Model file for the job. Use its own axes, mm. Face numbers are marked on the shaded views. A direction names the side the tool comes from. Coordinates: 2 decimals unless noted, no trailing zeros. Write each loop counter-clockwise with the first axis right and the second up, starting at its lowest first coordinate (ties: lowest second). Pieces come first, ordered by that corner, then holes. Notation, with made-up numbers: (80.5, -15) -> (88.5, -15) arc R16 ccw to (88.5, 8) -> close; hole circle Ø4 at (-5.5, 30.5). An arc over 180 degrees is marked (long way). Write item = value, one per line. Start each with the question number.
from build123d import *

# Parameters (mm, degrees)
BOSS_EXTRUDE1_DEPTH = 120
SKETCH2_R           = 40
BOSS_EXTRUDE2_DEPTH = 30
SKETCH4_R           = 60
BOSS_EXTRUDE3_DEPTH = 4
SHELL1_START        = 3
SHELL1_DEPTH        = 114
SHELL1_START_2      = 37.215764226
SHELL1_2_OUTLINE_R  = 37
SHELL1_2_DEPTH      = 34


with BuildPart() as part:
    # Sketch1 → Boss-Extrude1 (new body)
    with BuildSketch(Plane.XY):
        Polygon((40, 21.666666667), (-40, 75), (-40, -75), (40, -75), align=None)
    extrude(amount=BOSS_EXTRUDE1_DEPTH)

    # Sketch2 → Boss-Extrude2 (add)
    with BuildSketch(Plane(origin=(22.307692308, 33.461538462, 0), x_dir=(0, 0, -1), z_dir=(0.5547001962252291, 0.8320502943378437, 0))):
        with Locations(Location((-60, 26.810509484, 0), (0, 0, 90))):
            Circle(SKETCH2_R)
    extrude(amount=BOSS_EXTRUDE2_DEPTH)

    # Sketch4 → Boss-Extrude3 (add)
    with BuildSketch(Plane(origin=(38.948698194, 58.423047292, 0), x_dir=(0, 0, -1), z_dir=(0.5547001962252291, 0.8320502943378437, 0))):
        with Locations(Location((-60, 26.810509484, 0), (0, 0, 90))):
            Circle(SKETCH4_R)
    extrude(amount=BOSS_EXTRUDE3_DEPTH)

    # Shell1: read off the stored shape, not the designer's step
    # Shell1 outline → Shell1 (cut)
    with BuildSketch(Plane.XY.offset(SHELL1_START)):
        Polygon((-37, -72), (37, -72), (37, 20.061115391), (-37, 69.394448725), align=None)
    extrude(amount=SHELL1_DEPTH, mode=Mode.SUBTRACT)

    # Shell1 2 outline → Shell1 2 (cut)
    with BuildSketch(Plane(origin=(0, 0, 0), x_dir=(0.8320502943378438, -0.5547001962252289, 0), z_dir=(0.5547001962252289, 0.8320502943378438, 0)).offset(SHELL1_START_2)):
        with Locations((-26.810509484, -60)):
            Circle(SHELL1_2_OUTLINE_R)
    extrude(amount=SHELL1_2_DEPTH, mode=Mode.SUBTRACT)


solid = part.part
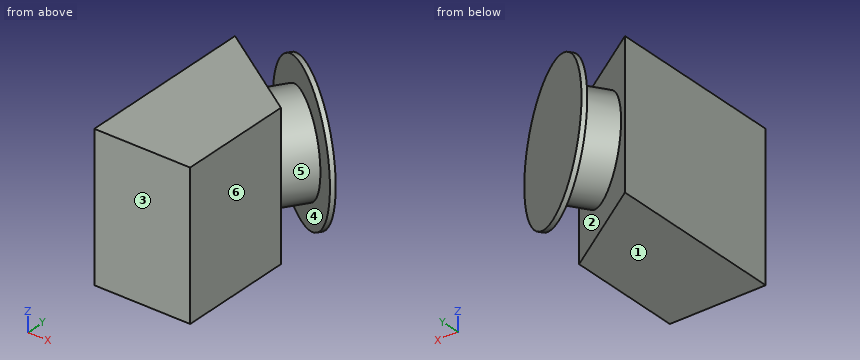
(1) Saw through at C-C (x = -26). State how many separate pieces and enclosed holes the cut face has, then the cut area to 3 significant figures.
(2) Saw through at A-A (z = 18). Give the cut face in (x, y).
(3) Saw through at D-D (z = 34). Give the cut face in (x, y).
(4) Drop flat-ended pins along their axis: pin 1 Ø22 at (x, y) = (0, 30) entering from -Z; pin 2 Ø1.5 at (x, z) = (49.5, 23) entering from +Y; pin 3 Ø10 at (x, y) = (48, -38) entering from +Z; pin 4 Ø8 at (y, z) = (-8, 65) entering from +X. Give the stop position or say it passes through.
(5) 3-axis set-ups, long thin cutter, end or side, ignore diameter. For the marked faces 1 and 2: which of +Z, -Z, +X, -X, +Y, -Y reach the whole face in a straight line?
(6) Drill centre lines: line 1 along Z through (x, y) = (13.5, -14.5); line 2 along X through (y, z) = (-37, 70.5); line 3 along Y through (x, z) = (-11.5, 99). Where is each one in solid material? Low to high.
(7) Mould opens along X. For the marked faces 3, 4, 5 and 6 say: released by +X, released by -X, zero draft, split by the parting line, or undercut.
(8) Saw through at B-B (y = -42). Give the cut face in (x, z), then the cut area to 3 significant figures.
Returned:
q1.separate_pieces = 2
q1.enclosed_holes = 1
q1.area = 1,980 mm2
q2.outline = (-40, -75) -> (40, -75) -> (40, 21.67) -> (-40, 75) -> close; (-19.01, 97.06) -> (52.29, 49.53) -> (54.51, 52.85) -> (-16.79, 100.39) -> close; hole (-37, -72) -> (37, -72) -> (37, 20.06) -> (-37, 69.39) -> close
q3.outline = (-40, -75) -> (40, -75) -> (40, 21.67) -> (25.29, 31.47) -> (41.93, 56.43) -> (61.63, 43.3) -> (63.85, 46.63) -> (-26.13, 106.62) -> (-28.35, 103.29) -> (-8.65, 90.16) -> (-25.29, 65.19) -> (-40, 75) -> close; hole (-37, -72) -> (37, -72) -> (37, 20.06) -> (20.24, 31.23) -> (39.1, 59.52) -> (-4.71, 88.73) -> (-23.57, 60.44) -> (-37, 69.39) -> close
q4.pin_1 = 0
q4.pin_2 = 56.7
q4.pin_3 = through
q4.pin_4 = 40
q5.face_1 = -Z, +X, -X, +Y, -Y
q5.face_2 = none
q6.line_1 = 0 to 3, 117 to 120
q6.line_2 = -40 to -37, 37 to 40
q6.line_3 = -75 to -72, 52.39 to 56, 92.06 to 96.86
q7.face_3 = zero draft
q7.face_4 = undercut
q7.face_5 = undercut
q7.face_6 = released by +X
q8.outline = (-40, 0) -> (40, 0) -> (40, 120) -> (-40, 120) -> close; hole (-37, 3) -> (37, 3) -> (37, 117) -> (-37, 117) -> close
q8.area = 1,160 mm2
